Source: CAD feature listing. Evaluate the final solid. Frame: model axes, mm. A direction names the side the tool comes from. Round coordinates to 2 decimals unless told otherwise and drop trailing zeros. Order: outer loops, then holes, each group sorted by start corner. A loop starts at its lowest first (then second) coordinate and runs counter-clockwise, first axis right, second up. Notation, with made-up numbers: (-2, -35) - (45, -35) arc R21 cw to (45, -29) - close; hole circle Ø9 at (-27.75, 61.25). An arc over 180 degrees is marked (long way). Use one line per item in the form item = value. Start each with the question number.
Q1. Ray query, line 1 (Z direction, x = 22, y = -8.5); line 2 (Z direction, x = 25, y = -0.75); line 3 (Z direction, x = -3, y = -7). Return the intervals inside material, ascending. Write a range as [from, to].
Q2. Draft query along X for faces 6 (the flat face through (14, -4, -17.5)), 7 (the flat face through (9, -3, -8)), 8 (the flat face through (13.649, -6, -11)), 9 (the flat face through (15.649, -1, 2)). Return one class per face: released by +X, released by -X, zero draft, split by the parting line, or undercut.
Q3. Cut plane A-A, the plane x = 19. Return the cut outline in (y, z), and give its area (3 significant figures).
Q4. Cut plane B-B, the plane z = -3.5. Return the cut outline in (x, y).
Q5. Pin query (flat end, axial travel): pin 1 Ø2 at (x, y) = (0.5, -5) entering from -Z; pin 2 Ø12.5 at (x, z) = (7, -8) entering from -Y; pin 3 Ø4 at (x, z) = (10.15, -3.5) entering from -Y. Return the tip coordinate at first contact, or that it passes through.
Q6. Set-up query: faces 1 (the flat face through (28.149, -6, -4)), 2 (the flat face through (15, -6, -4.5)), 3 (the flat face through (22, -1, 3.5)), 4 (the flat face through (30.149, -5, -4)), 5 (the flat face through (-9.851, -2.7, -0.8)). Return all of +Z, -Z, +X, -X, +Y, -Y with unobstructed straight access to the full face (end or side cutting, diameter ignored); none if empty.
Q7. Cut plane D-D, the plane z = -9.75. Return the cut outline in (x, y), and give its area (3 significant figures).
Q8. Cut plane C-C, the plane y = -1.75. Return the cut outline in (x, z).
from build123d import *

# Parameters (mm, degrees)
F1_DEPTH = 10
F0_R     = 2.5
F2_DEPTH = 3


with BuildPart() as f1:
    # F0 (on Front) → F1 (new body)
    with BuildSketch(Plane.XZ):
        Polygon((13.648517, -4.5), (13.648517, -17.5), (30.148517, -17.5), (30.148517, 9.5), (-9.851483, 9.5), (-9.851483, 7.5), (28.148517, 7.5), (28.148517, 3.5), (28.148517, 0), (28.148517, -15.5), (15.648517, -15.5), (15.648517, -4.5), align=None)
    extrude(amount=F1_DEPTH)

    # F0 (on Front) → F2 (join)
    with BuildSketch(Plane.XZ):
        Polygon((-9.851483, 7.5), (-9.851483, -17.5), (13.648517, -17.5), (13.648517, -4.5), (15.648517, -4.5), (15.648517, -15.5), (28.148517, -15.5), (28.148517, 0), (15.648517, 0), (15.648517, 3.5), (28.148517, 3.5), (28.148517, 7.5), align=None)
        with Locations((10.148517, -3.5)):
            Circle(F0_R, mode=Mode.SUBTRACT)
    extrude(amount=F2_DEPTH)


solid = f1.part
Completed:
q1.line_1 = [-17.5, -15.5], [7.5, 9.5]
q1.line_2 = [-17.5, 0], [3.5, 9.5]
q1.line_3 = [7.5, 9.5]
q2.face_6 = zero draft
q2.face_7 = undercut
q2.face_8 = released by -X
q2.face_9 = undercut
q3.outline = (-10, -17.5) - (0, -17.5) - (0, 0) - (-3, 0) - (-3, -15.5) - (-10, -15.5) - close; (-10, 7.5) - (-3, 7.5) - (-3, 3.5) - (0, 3.5) - (0, 9.5) - (-10, 9.5) - close
q3.area = 98.5 mm2
q4.outline = (-9.85, -3) - (7.65, -3) - (7.65, 0) - (-9.85, 0) - close; (12.65, -3) - (28.15, -3) - (28.15, -10) - (30.15, -10) - (30.15, 0) - (12.65, 0) - close
q5.pin_1 = 7.5
q5.pin_2 = -3
q5.pin_3 = through
q6.face_1 = -Y
q6.face_2 = -X, -Y
q6.face_3 = +Y, -Y
q6.face_4 = +Z, -Z, +X, +Y, -Y
q6.face_5 = +Z, -Z, -X, +Y, -Y
q7.outline = (-9.85, -3) - (13.65, -3) - (13.65, -10) - (15.65, -10) - (15.65, -3) - (28.15, -3) - (28.15, -10) - (30.15, -10) - (30.15, 0) - (-9.85, 0) - close
q7.area = 148 mm2
q8.outline = (-9.85, -17.5) - (30.15, -17.5) - (30.15, 9.5) - (-9.85, 9.5) - close; hole circle Ø5 at (10.15, -3.5); hole (15.65, 0) - (28.15, 0) - (28.15, 3.5) - (15.65, 3.5) - close
